Design review of the part built by this model. Coordinates are the model's own, in mm. Face numbers are marked on the shaded views. A direction names the side the tool comes from. Coordinates: 2 decimals unless noted, no trailing zeros. Loops run counter-clockwise (first coordinate to the right, second up) from the corner with the lowest first, then second, coordinate; pieces in that order, holes last. Notation, with made-up numbers: M 87,-20 L 100,-20 A16 ccw 100,-10 Z; hole C 57,47.25 d1. An arc over 180 degrees is marked long. Answer as CSV lines item,"result". Start each with the question number.
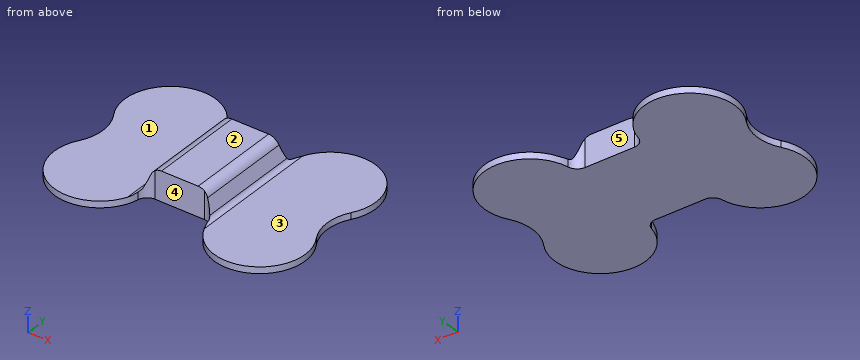
from build123d import *

# Parameters (mm, degrees)
BOSS_EXTRUDE1_DEPTH     = 27.56
CUT_EXTRUDE1_DEPTH      = 149.090525018
CUT_EXTRUDE1_DEPTH_BACK = 149.090525018


with BuildPart() as part:
    # Sketch1 → Boss-Extrude1 (new body)
    with BuildSketch(Plane.XY):
        with BuildLine():
            Line((22.96117968, 44), (-22.96117968, 44))
            ThreePointArc((-22.96117968, 44), (-29.323269783, 46.284832502), (-32.778097836, 52.095238095))
            ThreePointArc((-32.778097836, 52.095238095), (-89.927364847, 83.601091069), (-110.70300535, 21.738095238))
            ThreePointArc((-110.70300535, 21.738095238), (-104.55417528, 0), (-110.70300535, -21.738095238))
            ThreePointArc((-110.70300535, -21.738095238), (-89.927364847, -83.601091069), (-32.778097836, -52.095238095))
            ThreePointArc((-32.778097836, -52.095238095), (-29.323269783, -46.284832502), (-22.96117968, -44))
            Line((-22.96117968, -44), (22.96117968, -44))
            ThreePointArc((22.96117968, -44), (29.323269783, -46.284832502), (32.778097836, -52.095238095))
            ThreePointArc((32.778097836, -52.095238095), (89.927364847, -83.601091069), (110.70300535, -21.738095238))
            ThreePointArc((110.70300535, -21.738095238), (104.55417528, 0), (110.70300535, 21.738095238))
            ThreePointArc((110.70300535, 21.738095238), (89.927364847, 83.601091069), (32.778097836, 52.095238095))
            ThreePointArc((32.778097836, 52.095238095), (29.323269783, 46.284832502), (22.96117968, 44))
        make_face()
    extrude(amount=BOSS_EXTRUDE1_DEPTH)

    # Sketch2 → Cut-Extrude1 (cut, two sides: drawn at the far end of the back side and taken through both)
    with BuildSketch(Plane(origin=(0, 0, 0), x_dir=(1, 0, 0), z_dir=(0, 1, 0)).offset(-CUT_EXTRUDE1_DEPTH_BACK)):
        with BuildLine():
            Line((117, -6), (35.767564174, -6))
            ThreePointArc((35.767564174, -6), (32.945610035, -6.872461407), (31.108474327, -9.185370066))
            Line((31.108474327, -9.185370066), (26.433179694, -21.189259868))
            ThreePointArc((26.433179694, -21.189259868), (22.758908279, -25.815077185), (17.115, -27.56))
            Line((17.115, -27.56), (117, -27.56))
            Line((117, -27.56), (117, -6))
        make_face()
        with BuildLine():
            Line((-117, -27.56), (-117, -6))
            Line((-117, -6), (-35.767564174, -6))
            ThreePointArc((-35.767564174, -6), (-32.945610035, -6.872461407), (-31.108474327, -9.185370066))
            Line((-31.108474327, -9.185370066), (-26.433179694, -21.189259868))
            ThreePointArc((-26.433179694, -21.189259868), (-22.758908279, -25.815077185), (-17.115, -27.56))
            Line((-17.115, -27.56), (-117, -27.56))
        make_face()
    extrude(amount=CUT_EXTRUDE1_DEPTH + CUT_EXTRUDE1_DEPTH_BACK, mode=Mode.SUBTRACT)


solid = part.part
Item 1: For the marked faces 1 and 2, list the 3-axis set-ups (+Z, -Z, +X, -X, +Y, -Y) from which the entire face can be reached by the end or side of a thin tool; tool diameter is ignored.
Item 2: Add section D-D (x = -74.5). Give the boundary of the cut face in (y, z), plus the area to 3 significant figures.
Item 3: For line 1 along Z through (x, y) = (-41.5, -0.5); line 2 along Y through (x, z) = (-5, 17.75); line 3 along X through (y, z) = (68, 3.75), list the stretches that pass through material, from the lowest coordinate up. Write a range as from..to.
Item 4: Add section B-B (y = -3.5). Give the boundary of the cut face in (x, z) (3 decimals).
Item 5: For pin 1 (14 mm diameter, centred on x = -6.5, z = 9, fed in from -Y); pin 2 (5 mm diameter, centred on x = -24, z = 16.5, fed in from +Y); pin 3 (24.5 mm diameter, centred on x = 96, y = -18, fed in from +Z), all flat-tipped, find the tip position at first contact; note any pin that passes through.
Item 6: Add section C-C (x = -4.5). Give the boundary of the cut face in (y, z).
Item 7: Mouldability with a two-part tool opening along X and no side actions: class the marked faces 3, 4 and 5 as released by +X, released by -X, zero draft, split by the parting line, or undercut.
Item 8: Add section A-A (z = 3.5). Give the boundary of the cut face in (x, y), plus the area to 3 significant figures.
Response:
1,face 1,"+Z, -X, +Y, -Y"
1,face 2,"+Z, +X, -X, +Y, -Y"
2,outline,"M -86.5,0 L 86.5,0 L 86.5,6 L -86.5,6 Z"
2,area,"1,040 mm²"
3,line 1,"0..6"
3,line 2,"-44..44"
3,line 3,"-109.57..-39.43, 39.43..109.57"
4,outline,"M -104.702,0 L 104.702,0 L 104.702,6 L 35.768,6 A5 cw 31.108,9.185 L 26.433,21.189 A10 ccw 17.115,27.56 L -17.115,27.56 A10 ccw -26.433,21.189 L -31.108,9.185 A5 cw -35.768,6 L -104.702,6 Z"
5,pin 1,"y = -44"
5,pin 2,"y = 44.65"
5,pin 3,"z = 6"
6,outline,"M -44,0 L 44,0 L 44,27.56 L -44,27.56 Z"
7,face 3,"zero draft"
7,face 4,"undercut"
7,face 5,"undercut"
8,outline,"M -110.7,-21.74 A42.5 ccw long -32.78,-52.1 A10 cw -22.96,-44 L 22.96,-44 A10 cw 32.78,-52.1 A42.5 ccw long 110.7,-21.74 A41.5 cw 110.7,21.74 A42.5 ccw long 32.78,52.1 A10 cw 22.96,44 L -22.96,44 A10 cw -32.78,52.1 A42.5 ccw long -110.7,21.74 A41.5 cw Z"
8,area,"30,900 mm²"
